The drawing under review shows one solid part. Ordinate dimensions are in mm from its lowest x, y, z. A direction names the side the tool comes from. Round coordinates to 2 decimals unless told otherwise and drop trailing zeros. Loops run counter-clockwise (first coordinate to the right, second up) from the corner with the lowest first, then second, coordinate; pieces in that order, holes last. Notation, with made-up numbers: M 47,-39.5 L 53,-39.5 A15 ccw 53,-27.5 Z; hole C 17,41.25 d11. An arc over 180 degrees is marked long. Use a Markdown table: item, result.
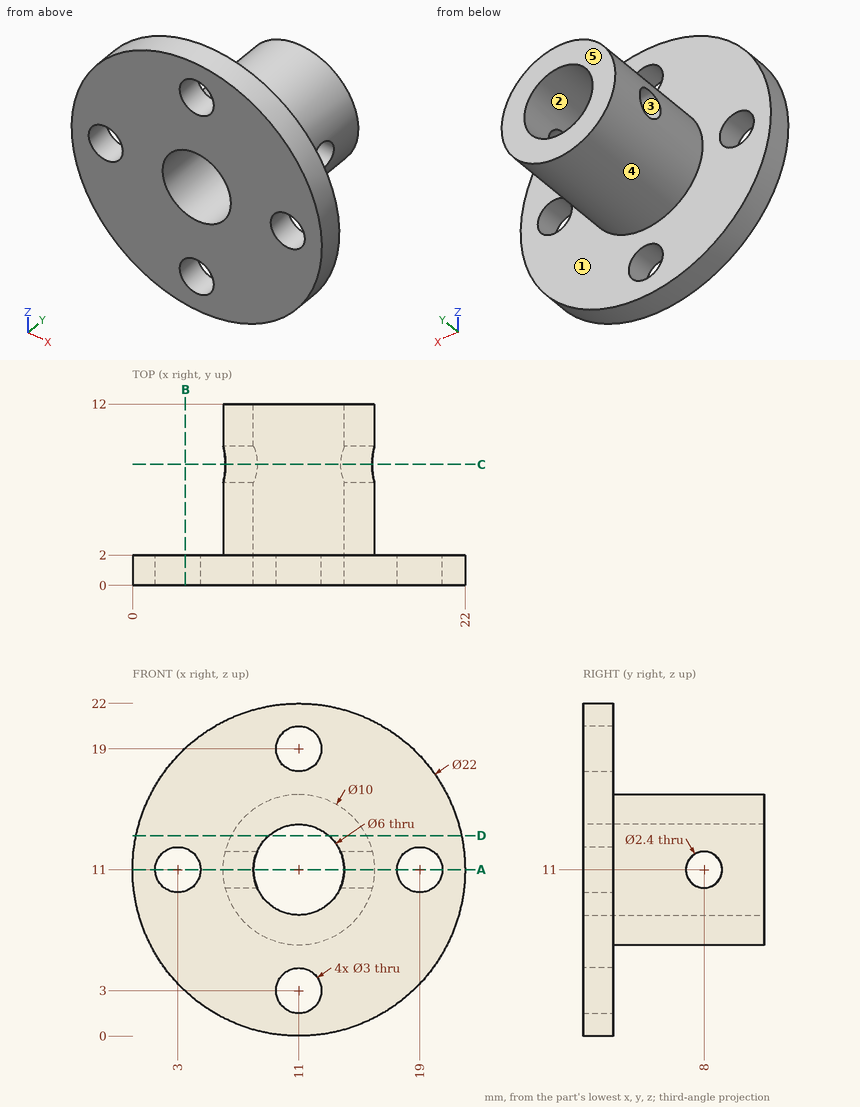
1. Take a section at D-D on z = 13.25. Give the boundary of the cut face in (x, y), and give its area (3 significant figures).
Check values:
| item | result |
|---|---|
| outline | M 0.23,0 L 9.02,0 L 9.02,12 L 6.53,12 L 6.53,2 L 0.23,2 Z; M 12.98,0 L 21.77,0 L 21.77,2 L 15.47,2 L 15.47,12 L 12.98,12 Z |
| area | 84.7 mm² |
2. The part is to be moulded in two halves that separate along Z. For the marked faces 3, 4 and 5, say which applies: pulls with the +Z half, pulls with the -Z half, needs draft (parallel to the pull), parting line crosses it, or undercut.
Check values:
| item | result |
|---|---|
| face 3 | undercut |
| face 4 | parting line crosses it |
| face 5 | needs draft |
3. Take a section at A-A on z = 11. Give the boundary of the cut face in (x, y), and give its area (3 significant figures).
Check values:
| item | result |
|---|---|
| outline | M 0,0 L 1.5,0 L 1.5,2 L 0,2 Z; M 4.5,0 L 8,0 L 8,6.8 L 6,6.8 L 6,2 L 4.5,2 Z; M 6,9.2 L 8,9.2 L 8,12 L 6,12 Z; M 14,0 L 17.5,0 L 17.5,2 L 16,2 L 16,6.8 L 14,6.8 Z; M 14,9.2 L 16,9.2 L 16,12 L 14,12 Z; M 20.5,0 L 22,0 L 22,2 L 20.5,2 Z |
| area | 50.4 mm² |
4. Insertion check: pin 1 (5 mm diameter, centred on y = 2.5, z = 2.5, fed in from -X); pin 2 (5.5 mm diameter, centred on x = 11, z = 11, fed in from +Y); pin 3 (1.5 mm diameter, centred on y = 2.5, z = 10, fed in from -X); pin 4 (11 mm diameter, centred on x = 8.5, z = 9.5, fed in from +Y). Each pin has a flat end and moves straight along its axis. Give the tip position at first contact, or say it passes through.
Check values:
| item | result |
|---|---|
| pin 1 | stops at x = 1.81 |
| pin 2 | passes through |
| pin 3 | stops at x = 0.01 |
| pin 4 | stops at y = 12 |
5. Take a section at B-B on x = 3.5. Give the boundary of the cut face in (y, z), and give its area (3 significant figures).
Check values:
| item | result |
|---|---|
| outline | M 0,2.95 L 2,2.95 L 2,9.59 L 0,9.59 Z; M 0,12.41 L 2,12.41 L 2,19.05 L 0,19.05 Z |
| area | 26.5 mm² |
6. Take a section at C-C on y = 8. Give the boundary of the cut face in (x, z).
Check values:
| item | result |
|---|---|
| outline | M 6.15,9.8 A5 ccw 15.85,9.8 L 13.75,9.8 A3 cw 8.25,9.8 Z; M 6.15,12.2 L 8.25,12.2 A3 cw 13.75,12.2 L 15.85,12.2 A5 ccw Z |
7. Wall thickness on line 1 along X through (y, z) = (0.95, 11); line 2 along Y through (x, z) = (15.25, 11); line 3 along Y through (x, z) = (11.25, 16.5): over which ranges is each line inside the solid? List them lowest first. Write a range as from..to.
Check values:
| item | result |
|---|---|
| line 1 | x = 0..1.5, 4.5..8, 14..17.5, 20.5..22 |
| line 2 | y = 0..6.8, 9.2..12 |
| line 3 | y = 0..2 |
8. Machinability: for the marked faces 1 and 2, which of the approach directions +Z, -Z, +X, -X, +Y, -Y give a long, thin tool a straight path to every point of the face, cutting with its end or side? Answer none if there is none.
Check values:
| item | result |
|---|---|
| face 1 | +Y |
| face 2 | +Y, -Y |
